Build history of the part. All positions in model axes, mm. A direction names the side the tool comes from. Round coordinates to 2 decimals unless told otherwise and drop trailing zeros. Order: outer loops, then holes, each group sorted by start corner. A loop starts at its lowest first (then second) coordinate and runs counter-clockwise, first axis right, second up. Notation, with made-up numbers: (53.5, 30) -> (78.5, 30) arc R26 ccw to (78.5, 44) -> close; hole circle Ø3 at (87, 85). An arc over 180 degrees is marked (long way). Answer as CSV lines item,"result". Start each with the question number.
```python
from build123d import *

# Parameters (mm, degrees)
F1_DEPTH = 25
F2_R     = 6
F2_R_2   = 3
F3_DEPTH = 45.001
F4_R     = 6
F5_DEPTH = 8.8
F6_R     = 6
F7_DEPTH = 8.5
F8_R     = 4


with BuildPart() as f1:
    # F0 (on Front) → F1 (new body)
    with BuildSketch(Plane.XZ):
        Polygon((0, 15), (0, 0), (80, 0), (80, 45), (0, 45), (0, 30), (65, 30), (65, 15), align=None)
    extrude(amount=F1_DEPTH)

    # F2 (on face) → F3 (cut, through all)
    with BuildSketch(Plane.XY.offset(45)):
        with Locations((40, -12.5)):
            Circle(F2_R)
        with Locations((8, -12.5)):
            Circle(F2_R_2)
        with Locations((25, -12.5)):
            Circle(F2_R_2)
        with Locations((72, -12.5)):
            Circle(F2_R_2)
    extrude(amount=-F3_DEPTH, mode=Mode.SUBTRACT)

    # F4 (on face) → F5 (cut)
    with BuildSketch(Plane(origin=(0, 0, 30), x_dir=(1, 0, 0), z_dir=(0, 0, -1))):
        Polygon((35.092523, 4), (44.907477, 4), (49.814955, 12.5), (44.907477, 21), (35.092523, 21), (30.185045, 12.5), align=None)
        with Locations((40, 12.5)):
            Circle(F4_R, mode=Mode.SUBTRACT)
    extrude(amount=-F5_DEPTH, mode=Mode.SUBTRACT)

    # F6 (on face) → F7 (cut)
    with BuildSketch(Plane.XY.offset(15)):
        Polygon((35.092523, -21), (44.907477, -21), (49.814955, -12.5), (44.907477, -4), (35.092523, -4), (30.185045, -12.5), align=None)
        with Locations((40, -12.5)):
            Circle(F6_R, mode=Mode.SUBTRACT)
    extrude(amount=-F7_DEPTH, mode=Mode.SUBTRACT)

    # F8
    f8_edges = [f1.edges().sort_by_distance(p)[0] for p in [
        (80, -12.5, 45),
        (80, -12.5, 0),
        (65, -12.5, 30),
        (65, -12.5, 15),
    ]]
    fillet(f8_edges, radius=F8_R)


solid = f1.part
```
Q1. Slice it at B-B, the plane z = 36. Write the cut outline in (x, y), plus the area to 3 significant figures.
Q2. Flat gauge pin, fed straight in: pin 1 Ø3.5 at (x, y) = (8, -12.5) entering from -Z. Where does the tip first touch, or does it go through?
Q3. Slice it at D-D, the plane x = 8. Write the cut outline in (y, z), plus the area to 3 significant figures.
Q4. Slice it at A-A, the plane x = 40. Write the cut outline in (y, z), plus the area to 4 significant figures.
Q5. Which spindle directions (+Z, -Z, +X, -X, +Y, -Y) get a long thin tool onto all of the face, cutting with end or side? Do faces 5 (the face through (35.58, -8.44, 41.94)), 6 (the face through (47.396, -8.31, 10.81)), 7 (the face through (31, -10, 15)). Say none if no direction does.
Q6. Probe L1, parallel to Z at x = 60, y = -17; L2, parallel to Z at x = 31, y = -13.5; L3, parallel to Y at x = 25, z = 41. List the from-to ranges inside material, lowest first.
Q7. Two-plate mould, pull along Z, no slides. Class faces 1 (the face through (46.4, -12.4, 6.5)), 2 (the face through (39, -25, 33)), 3 (the face through (78.859, -12.675, 43.797)), 4 (the face through (78.797, -12.675, 1.141)): +Z half, -Z half, draft (parallel to the pull), parting line (faces both ways), or undercut.
Q8. Slice it at C-C, the plane z = 22.5. Write the cut outline in (x, y).
Solutions:
1,outline,"(0, -25) -> (80, -25) -> (80, 0) -> (0, 0) -> close; hole circle Ø6 at (8, -12.5); hole circle Ø6 at (25, -12.5); hole (30.19, -12.5) -> (35.09, -21) -> (44.91, -21) -> (49.81, -12.5) -> (44.91, -4) -> (35.09, -4) -> close; hole circle Ø6 at (72, -12.5)"
1,area,"1,660 mm2"
2,pin 1,"passes through"
3,outline,"(-25, 0) -> (-15.5, 0) -> (-15.5, 15) -> (-25, 15) -> close; (-25, 30) -> (-15.5, 30) -> (-15.5, 45) -> (-25, 45) -> close; (-9.5, 0) -> (0, 0) -> (0, 15) -> (-9.5, 15) -> close; (-9.5, 30) -> (0, 30) -> (0, 45) -> (-9.5, 45) -> close"
3,area,"570 mm2"
4,outline,"(-25, 0) -> (-18.5, 0) -> (-18.5, 6.5) -> (-21, 6.5) -> (-21, 15) -> (-25, 15) -> close; (-25, 30) -> (-21, 30) -> (-21, 38.8) -> (-18.5, 38.8) -> (-18.5, 45) -> (-25, 45) -> close; (-6.5, 0) -> (0, 0) -> (0, 15) -> (-4, 15) -> (-4, 6.5) -> (-6.5, 6.5) -> close; (-6.5, 38.8) -> (-4, 38.8) -> (-4, 30) -> (0, 30) -> (0, 45) -> (-6.5, 45) -> close"
4,area,"303.5 mm2"
5,face 5,"+Z, -Z"
5,face 6,"none"
5,face 7,"-X, +Y, -Y"
6,L1,"z = 0 to 15, 30 to 45"
6,L2,"z = 0 to 6.5, 38.8 to 45"
6,L3,"y = -25 to -15.5, -9.5 to 0"
7,face 1,"undercut"
7,face 2,"draft"
7,face 3,"+Z half"
7,face 4,"-Z half"
8,outline,"(65, -25) -> (80, -25) -> (80, 0) -> (65, 0) -> close; hole circle Ø6 at (72, -12.5)"
